Can you work these out from the model? Positions are in its coordinate system, mm. A direction names the side the tool comes from. Round coordinates to 2 decimals unless told otherwise and drop trailing zeros. Loops run counter-clockwise (first coordinate to the right, second up) from the corner with the lowest first, then second, coordinate; pieces in that order, holes last.
```python
from build123d import *

# Parameters (mm, degrees)
SKETCH1_W                 = 130
SKETCH1_H                 = 125
BOSS_EXTRUDE1_DEPTH       = 5
SKETCH2_R                 = 1.75
SKETCH2_R_2               = 12.65
CUT_EXTRUDE1_DEPTH        = 10
SKETCH4_R                 = 2.15
CUT_EXTRUDE3_DEPTH        = 10
BOSS_EXTRUDE2_DEPTH       = 2
MIRROR7_COPY_1_SKETCH_R   = 1.75
MIRROR7_COPY_1_SKETCH_R_2 = 12.65
MIRROR7_COPY_1_DEPTH      = 10
MIRROR7_COPY_2_DEPTH      = 2
SKETCH10_R                = 2.15
CUT_EXTRUDE8_DEPTH        = 91.311959341
SKETCH11_R                = 2.65
CUT_EXTRUDE9_DEPTH        = 0.5
CUT_EXTRUDE10_DEPTH       = 91.444734507
CUT_EXTRUDE11_DEPTH       = 91.444734507


with BuildPart() as part:
    # Sketch1 → Boss-Extrude1 (new body)
    with BuildSketch(Plane(origin=(0, 0, 0), x_dir=(1, 0, 0), z_dir=(0, 1, 0))):
        Rectangle(SKETCH1_W, SKETCH1_H)
    extrude(amount=BOSS_EXTRUDE1_DEPTH)

    # Sketch2 → Cut-Extrude1 (cut)
    with BuildSketch(Plane(origin=(0, 5, 0), x_dir=(1, 0, 0), z_dir=(0, 1, 0))):
        with Locations(Location((-61, -52.5, 0), (0, 0, 270))):
            Circle(SKETCH2_R)
        with Locations(Location((-36, -52.5, 0), (0, 0, 270))):
            Circle(SKETCH2_R)
        with Locations(Location((-36, -10.5, 0), (0, 0, 270))):
            Circle(SKETCH2_R)
        with Locations(Location((-61, -10.5, 0), (0, 0, 270))):
            Circle(SKETCH2_R)
        with Locations(Location((-45.5, -31.5, 0), (0, 0, 270))):
            Circle(SKETCH2_R_2)
    cut_extrude1 = extrude(amount=-CUT_EXTRUDE1_DEPTH, mode=Mode.SUBTRACT)

    # Mirror3: Cut-Extrude1 across plane
    add(cut_extrude1.mirror(Plane.ZY), mode=Mode.SUBTRACT)

    # Sketch4 → Cut-Extrude3 (cut)
    with BuildSketch(Plane(origin=(0, 5, 0), x_dir=(1, 0, 0), z_dir=(0, 1, 0))):
        with Locations(Location((0, 47.5, 0), (0, 0, 270))):
            Circle(SKETCH4_R)
        with Locations(Location((12.049810205, 55, 0), (0, 0, 270))):
            Circle(SKETCH4_R)
        with Locations(Location((-12.049810205, 55, 0), (0, 0, 270))):
            Circle(SKETCH4_R)
    extrude(amount=-CUT_EXTRUDE3_DEPTH, mode=Mode.SUBTRACT)

    # Sketch5 → Boss-Extrude2 (add)
    with BuildSketch(Plane.XZ):
        Polygon((-65, 58.7), (-65, 56.7), (-31.6, 56.7), (-31.6, 6.3), (-65, 6.3), (-65, 4.3), (-29.6, 4.3), (-29.6, 58.7), align=None)
    boss_extrude2 = extrude(amount=BOSS_EXTRUDE2_DEPTH)

    # Mirror5: Boss-Extrude2 across plane
    add(boss_extrude2.mirror(Plane.ZY))

    # Mirror7: Cut-Extrude1, Boss-Extrude2 across plane
    add(cut_extrude1.mirror(Plane.XY.offset(-1.9)), mode=Mode.SUBTRACT)
    add(boss_extrude2.mirror(Plane.XY.offset(-1.9)))

    # Mirror7 copy 1 sketch → Mirror7 copy 1 (cut)
    with BuildSketch(Plane(origin=(0, 5, -3.8), x_dir=(-1, 0, 0), z_dir=(0, 1, 0))):
        with Locations(Location((-61, -52.5, 0), (0, 0, 270))):
            Circle(MIRROR7_COPY_1_SKETCH_R)
        with Locations(Location((-36, -52.5, 0), (0, 0, 270))):
            Circle(MIRROR7_COPY_1_SKETCH_R)
        with Locations(Location((-36, -10.5, 0), (0, 0, 270))):
            Circle(MIRROR7_COPY_1_SKETCH_R)
        with Locations(Location((-61, -10.5, 0), (0, 0, 270))):
            Circle(MIRROR7_COPY_1_SKETCH_R)
        with Locations(Location((-45.5, -31.5, 0), (0, 0, 270))):
            Circle(MIRROR7_COPY_1_SKETCH_R_2)
    extrude(amount=-MIRROR7_COPY_1_DEPTH, mode=Mode.SUBTRACT)

    # Mirror7 copy 2 sketch → Mirror7 copy 2 (add)
    with BuildSketch(Plane(origin=(0, 0, -3.8), x_dir=(-1, 0, 0), z_dir=(0, -1, 0))):
        Polygon((-65, 58.7), (-65, 56.7), (-31.6, 56.7), (-31.6, 6.3), (-65, 6.3), (-65, 4.3), (-29.6, 4.3), (-29.6, 58.7), align=None)
    extrude(amount=MIRROR7_COPY_2_DEPTH)

    # Sketch10 → Cut-Extrude8 (cut, through all)
    with BuildSketch(Plane(origin=(0, 0, 0), x_dir=(-1, 0, 0), z_dir=(0, -1, 0))):
        with Locations(Location((-24.17, -42.03, 0), (0, 0, 90))):
            Circle(SKETCH10_R)
        with Locations(Location((24.17, -42.03, 0), (0, 0, 90))):
            Circle(SKETCH10_R)
        with Locations(Location((-8.73, 9.6, 0), (0, 0, 90))):
            Circle(SKETCH10_R)
        with Locations(Location((19.29, 9.6, 0), (0, 0, 90))):
            Circle(SKETCH10_R)
        with Locations(Location((-24.17, 33.11, 0), (0, 0, 90))):
            Circle(SKETCH10_R)
        with Locations(Location((24.17, 40.6, 0), (0, 0, 90))):
            Circle(SKETCH10_R)
    extrude(amount=-CUT_EXTRUDE8_DEPTH, mode=Mode.SUBTRACT)

    # Sketch11 → Cut-Extrude9 (cut)
    with BuildSketch(Plane.XZ):
        with Locations(Location((-12.049810205, -55, 0), (0, 0, 270))):
            Circle(SKETCH11_R)
        with Locations(Location((0, -47.5, 0), (0, 0, 270))):
            Circle(SKETCH11_R)
        with Locations(Location((12.049810205, -55, 0), (0, 0, 270))):
            Circle(SKETCH11_R)
        with Locations(Location((-24.17, -40.6, 0), (0, 0, 270))):
            Circle(SKETCH11_R)
        with Locations(Location((24.17, -33.11, 0), (0, 0, 270))):
            Circle(SKETCH11_R)
        with Locations(Location((8.73, -9.6, 0), (0, 0, 270))):
            Circle(SKETCH11_R)
        with Locations(Location((-19.29, -9.6, 0), (0, 0, 270))):
            Circle(SKETCH11_R)
        with Locations(Location((-24.17, 42.03, 0), (0, 0, 270))):
            Circle(SKETCH11_R)
        with Locations(Location((24.17, 42.03, 0), (0, 0, 270))):
            Circle(SKETCH11_R)
        with Locations(Location((-61, -14.3, 0), (0, 0, 270))):
            Circle(SKETCH11_R)
        with Locations(Location((-36, -14.3, 0), (0, 0, 270))):
            Circle(SKETCH11_R)
        with Locations(Location((-61, -56.3, 0), (0, 0, 270))):
            Circle(SKETCH11_R)
        with Locations(Location((-36, -56.3, 0), (0, 0, 270))):
            Circle(SKETCH11_R)
        with Locations(Location((36, -56.3, 0), (0, 0, 270))):
            Circle(SKETCH11_R)
        with Locations(Location((61, -56.3, 0), (0, 0, 270))):
            Circle(SKETCH11_R)
        with Locations(Location((36, -14.3, 0), (0, 0, 270))):
            Circle(SKETCH11_R)
        with Locations(Location((61, -14.3, 0), (0, 0, 270))):
            Circle(SKETCH11_R)
        with Locations(Location((36, 10.5, 0), (0, 0, 270))):
            Circle(SKETCH11_R)
        with Locations(Location((61, 10.5, 0), (0, 0, 270))):
            Circle(SKETCH11_R)
        with Locations(Location((61, 52.5, 0), (0, 0, 270))):
            Circle(SKETCH11_R)
        with Locations(Location((36, 52.5, 0), (0, 0, 270))):
            Circle(SKETCH11_R)
        with Locations(Location((-36, 52.5, 0), (0, 0, 270))):
            Circle(SKETCH11_R)
        with Locations(Location((-36, 10.5, 0), (0, 0, 270))):
            Circle(SKETCH11_R)
        with Locations(Location((-61, 10.5, 0), (0, 0, 270))):
            Circle(SKETCH11_R)
        with Locations(Location((-61, 52.5, 0), (0, 0, 270))):
            Circle(SKETCH11_R)
    extrude(amount=-CUT_EXTRUDE9_DEPTH, mode=Mode.SUBTRACT)

    # Sketch12 → Cut-Extrude10 (cut, through all)
    with BuildSketch(Plane(origin=(0, 5, 0), x_dir=(1, 0, 0), z_dir=(0, 1, 0))):
        Polygon((-2.363095604, -26.45), (-20.17, 1.845056316), (-20.17, -54.745056316), align=None)
        Polygon((17.806904396, 5.6), (-17.806904396, 5.6), (0, -22.695056316), align=None)
        Polygon((20.17, -54.745056316), (20.17, 1.845056316), (2.363095604, -26.45), align=None)
        Polygon((0, -30.204943684), (-17.806904396, -58.5), (17.806904396, -58.5), align=None)
    extrude(amount=-CUT_EXTRUDE10_DEPTH, mode=Mode.SUBTRACT)

    # Sketch13 → Cut-Extrude11 (cut, through all)
    with BuildSketch(Plane(origin=(0, 5, 0), x_dir=(1, 0, 0), z_dir=(0, 1, 0))):
        Polygon((-61, 1.9), (-61, -3.1), (-24.17, -3.1), (-24.17, 6.9), (-61, 6.9), align=None)
    cut_extrude11 = extrude(amount=-CUT_EXTRUDE11_DEPTH, mode=Mode.SUBTRACT)

    # Mirror9: Cut-Extrude11 across plane
    add(cut_extrude11.mirror(Plane.ZY), mode=Mode.SUBTRACT)


solid = part.part
```
(1) Suppose I cut it at B-B (z = 35.5). Give the number of separate pieces and of enclosed holes in the cut face, then the cut area to 3 significant figures.
(2) If I drill on line 1 (X direction, y = 2.8, z = -14.3); line 2 (Z direction, x = -43, y = -0.75); line 3 (X direction, y = -0.75, z = -19.5), over which ranges is the centre line in solid material (lowest first)?
(3) Suppose I cut it at A-A (z = -33.11). Write out the boundary of the cut face in (x, y).
(4) For pin 1 (2 mm diameter, centred on x = 61, z = -14.3, fed in from -Y); pin 2 (5 mm diameter, centred on x = -19.29, z = -9.6, fed in from -Y); pin 3 (0.6 mm diameter, centred on y = -0.5, z = 29, fed in from -X); pin 4 (12 mm diameter, centred on x = 9, z = -20, fed in from -Y), each with a flat end and sliding along its axis, tell me the tip position at first contact or that it passes through.
(5) Which directions (+Z, -Z, +X, -X, +Y, -Y) give clear straight access to the entire face, cutting with the end or side of a thin tool? Please do faces 1 (the flat face through (-63, 0.5, 10)), 2 (the flat face through (0, 3, 58.5)), 3 (the flat face through (30, -2, -35)).
(6) We'd pull the mould along X, two halves only. Please class faces 4 (the flat face through (-65, 3, -1)), 5 (the flat face through (59, 0, 31)), 6 (the cylindrical face through (-16.66, 0.25, -9.26)): released by +X, released by -X, zero draft, split by the parting line, or undercut.
Check result:
1. separate pieces: 6
1. enclosed holes: 0
1. area: 264 mm2
2. line 1: x = -65 to -62.75, -59.25 to -37.75, -34.25 to 34.25, 37.75 to 59.25, 62.75 to 65
2. line 2: z = -62.5 to -60.5, -10.1 to -8.1, 4.3 to 6.3, 56.7 to 58.7
2. line 3: x = -31.6 to -29.6, 29.6 to 31.6
3. outline: (-65, 0) - (-57.96, 0) - (-57.96, 5) - (-65, 5) - close; (-33.04, 0) - (-31.6, 0) - (-31.6, -2) - (-29.6, -2) - (-29.6, 0) - (21.52, 0) - (21.52, 0.5) - (22.02, 0.5) - (22.02, 5) - (-33.04, 5) - close; (26.32, 0.5) - (26.82, 0.5) - (26.82, 0) - (29.6, 0) - (29.6, -2) - (31.6, -2) - (31.6, 0) - (33.04, 0) - (33.04, 5) - (26.32, 5) - close; (57.96, 0) - (65, 0) - (65, 5) - (57.96, 5) - close
4. pin 1: passes through
4. pin 2: stops at y = 0.5
4. pin 3: stops at x = -31.6
4. pin 4: stops at y = 0
5. face 1: -Y
5. face 2: +Y, -Y
5. face 3: +Z, -Z, +X, -X, -Y
6. face 4: released by -X
6. face 5: zero draft
6. face 6: undercut
